Work out the finished part from the listing and answer in its coordinate system (mm). A direction names the side the tool comes from. Coordinates: 2 decimals unless noted, no trailing zeros. Order: outer loops, then holes, each group sorted by start corner. A loop starts at its lowest first (then second) coordinate and runs counter-clockwise, first axis right, second up. Notation, with made-up numbers: (11, -27.5) - (59, -27.5) arc R7 cw to (59, -18.5) - close; hole circle Ø10 at (21.25, -28). An arc over 180 degrees is marked (long way). Answer as a JSON object with one key per item and string values. Group by question number.
1) Section A-A (y = 30) is taken. Give the vertices of the cut face in (x, z).
2) A tool of negligible diameter and unlimited length cuts with its end or side. For faces 4 (the face through (0, -11, -1)), 5 (the face through (118, -13, 1)), 6 (the face through (106, -17, -1)), 7 (the face through (41, 7.115, 23)), from which of +Z, -Z, +X, -X, +Y, -Y can it reach the whole face along a straight path? Write none if from no direction.
3) Each of these flat-tipped pins is pushed along its axis until it touches: P1, Ø4, axis at x = 18, z = 20.5, coming from the +Y side; P2, Ø11, axis at y = 32, z = 19, coming from the -X side; P3, Ø5, axis at x = 59.5, z = -22, coming from the -Y side. Where does it stop, or does it pass through?
4) Find the intervals of material crossed by line 1 along Y through (x, z) = (36, -20.5); line 2 along X through (y, z) = (-24, 22.5); line 3 along Z through (x, y) = (64, 17), in increasing order.
5) Section C-C (x = 99) is taken. Give the vertices of the cut face in (y, z).
6) The mould has two halves that part along Z. Classify faces 1 (the face through (66, 17, -6)), 2 (the face through (92, 30, -23)), 3 (the face through (6, -17, -23)): released by +Z, released by -Z, zero draft, split by the parting line, or undercut.
7) Section B-B (z = 10) is taken. Give the vertices of the cut face in (x, y), plus the area to 3 significant figures.
8) Section D-D (y = 23) is taken. Give the vertices of the cut face in (x, z), plus the area to 3 significant figures.
from build123d import *

# Parameters (mm, degrees)
BOSS_EXTRUDE1_DEPTH     = 41
BOSS_EXTRUDE2_DEPTH     = 6
CUT_EXTRUDE1_DEPTH      = 132.512198268
CUT_EXTRUDE1_DEPTH_BACK = 132.512198268
SKETCH2_R               = 6
FILLET1_R               = 12


with BuildPart() as part:
    # Sketch1 → Boss-Extrude1 (new, symmetric)
    with BuildSketch(Plane.XY):
        with BuildLine():
            Line((118, 3.645195256), (118, 7.115183246))
            Line((118, 7.115183246), (118, 27.115183246))
            ThreePointArc((118, 27.115183246), (108.100505063, 31.215688309), (104, 41.115183246))
            Line((104, 41.115183246), (92, 41.115183246))
            Line((92, 41.115183246), (92, 19.115183246))
            ThreePointArc((92, 19.115183246), (88.485281374, 10.629901872), (80, 7.115183246))
            Line((80, 7.115183246), (0, 7.115183246))
            Line((0, 7.115183246), (0, 0))
            Line((0, 0), (0, -28.884816754))
            Line((0, -28.884816754), (12, -28.884816754))
            Line((12, -28.884816754), (12, -4.884816754))
            Line((12, -4.884816754), (106, -4.884816754))
            Line((106, -4.884816754), (106, -28.884816754))
            Line((106, -28.884816754), (118, -28.884816754))
            Line((118, -28.884816754), (118, 0))
            Line((118, 0), (118, 3.645195256))
        make_face()
        with BuildLine():
            Line((118, 27.115183246), (118, 7.115183246))
            Line((118, 7.115183246), (118, 3.645195256))
            ThreePointArc((118, 3.645195256), (120.497826292, 11.626423231), (127.1, 16.759691052))
            ThreePointArc((127.1, 16.759691052), (139.361179743, 26.29290272), (144, 41.115183246))
            Line((144, 41.115183246), (132, 41.115183246))
            ThreePointArc((132, 41.115183246), (127.899494937, 31.215688309), (118, 27.115183246))
        make_face()
    extrude(amount=BOSS_EXTRUDE1_DEPTH, both=True)

    # Sketch1_3 → Boss-Extrude2 (add, symmetric)
    with BuildSketch(Plane.XY):
        with BuildLine():
            Line((0, 7.115183246), (80, 7.115183246))
            ThreePointArc((80, 7.115183246), (88.485281374, 10.629901872), (92, 19.115183246))
            Line((92, 19.115183246), (92, 41.115183246))
            Line((92, 41.115183246), (0, 7.115183246))
        make_face()
    extrude(amount=BOSS_EXTRUDE2_DEPTH, both=True)

    # Sketch2 → Cut-Extrude1 (cut, two sides: drawn at the far end of the back side and taken through both)
    with BuildSketch(Plane(origin=(118, 0, 0), x_dir=(0, 0, -1), z_dir=(1, 0, 0)).offset(-CUT_EXTRUDE1_DEPTH_BACK)):
        with Locations((-29, -16.884816754)):
            Circle(SKETCH2_R)
        with Locations((29, -16.884816754)):
            Circle(SKETCH2_R)
    extrude(amount=CUT_EXTRUDE1_DEPTH + CUT_EXTRUDE1_DEPTH_BACK, mode=Mode.SUBTRACT)

    # Fillet1
    fillet1_edges = [part.edges().sort_by_distance(p)[0] for p in [
        (112, -28.884816754, -41),
        (6, -28.884816754, -41),
        (6, -28.884816754, 41),
        (112, -28.884816754, 41),
    ]]
    fillet(fillet1_edges, radius=FILLET1_R)


solid = part.part
Report:
{
 "1": {"outline": "(61.92, -6) - (92, -6) - (92, -41) - (109.49, -41) - (109.49, 41) - (92, 41) - (92, 6) - (61.92, 6) - close; (126.51, -41) - (141.5, -41) - (141.5, 41) - (126.51, 41) - close"},
 "2": {"face 4": "+Z, -Z, -X, +Y, -Y", "face 5": "+Z, -Z, +X, -Y", "face 6": "+Z, -Z, -Y", "face 7": "+Z, -X, +Y"},
 "3": {"P1": "stops at y = 7.12", "P2": "stops at x = 92", "P3": "stops at y = -4.88"},
 "4": {"line 1": "y = -4.88 to 7.12", "line 2": "x = 0 to 12, 106 to 118", "line 3": "z = -6 to 6"},
 "5": {"outline": "(-4.88, -41) - (41.12, -41) - (41.12, 41) - (-4.88, 41) - close"},
 "6": {"face 1": "released by -Z", "face 2": "zero draft", "face 3": "undercut"},
 "7": {"outline": "(0, -28.88) - (12, -28.88) - (12, -4.88) - (106, -4.88) - (106, -28.88) - (118, -28.88) - (118, 3.65) arc R14 cw to (127.1, 16.76) arc R26 ccw to (144, 41.12) - (132, 41.12) arc R14 cw to (104, 41.12) - (92, 41.12) - (92, 19.12) arc R12 cw to (80, 7.12) - (0, 7.12) - close", "area": "3,150 mm²"},
 "8": {"outline": "(42.98, -6) - (92, -6) - (92, -41) - (136.65, -41) - (136.65, 41) - (92, 41) - (92, 6) - (42.98, 6) - close", "area": "4,250 mm²"}
}
